from build123d import *

# Parameters (mm, degrees)
SKETCH1_W              = 36
SKETCH1_H              = 79.20150733
BOSS_EXTRUDE1_DEPTH    = 33.93
CUT_EXTRUDE1_REACH     = 65.368
SKETCH2_W              = 23.93
SKETCH2_H              = 8
SKETCH3_W              = 30.4
SKETCH3_H              = 7.2
CUT_EXTRUDE2_DEPTH     = 31.93
CUT_EXTRUDE3_START     = -3
CUT_EXTRUDE3_DEPTH     = 73.2
CUT_EXTRUDE4_REACH     = 55.961
BOSS_EXTRUDE2_REACH    = 57.168
LPATTERN1_COUNT        = 4
LPATTERN1_PITCH        = 16.8
LPATTERN1_COPY_1_REACH = 57.168
LPATTERN1_COPY_2_REACH = 57.168
LPATTERN1_COPY_3_REACH = 57.168
SKETCH7_W              = 36
SKETCH7_H              = 79.20150733
CUT_EXTRUDE5_DEPTH     = 2
FILLET1_R              = 1.5875
MOVE_START             = -34.93
MOVE_FACE1_OUTLINE_W   = 36
MOVE_FACE1_OUTLINE_H   = 63.20150733
MOVE_FACE1_DEPTH       = 1


# Read off the part's stored shape, not the designer's step: Move Face1
with BuildPart() as part:
    # Sketch1 → Boss-Extrude1 (new body)
    with BuildSketch(Plane.XY):
        Rectangle(SKETCH1_W, SKETCH1_H)
    extrude(amount=-BOSS_EXTRUDE1_DEPTH)

    # Sketch2 → Cut-Extrude1 (cut, up to next)
    with BuildSketch(Plane(origin=(18, 0, 0), x_dir=(0, 0, -1), z_dir=(1, 0, 0)), mode=Mode.PRIVATE) as cut_extrude1_sk1:
        with Locations((21.965, 35.600753665)):
            Rectangle(SKETCH2_W, SKETCH2_H)
    cut_extrude1_tool1 = extrude(cut_extrude1_sk1.sketch, amount=-CUT_EXTRUDE1_REACH, mode=Mode.PRIVATE) & part.part
    # Sketch2 → Cut-Extrude1 (cut, up to next)
    with BuildSketch(Plane(origin=(18, 0, 0), x_dir=(0, 0, -1), z_dir=(1, 0, 0)), mode=Mode.PRIVATE) as cut_extrude1_sk2:
        with Locations((21.965, -35.600753665)):
            Rectangle(SKETCH2_W, SKETCH2_H)
    cut_extrude1_tool2 = extrude(cut_extrude1_sk2.sketch, amount=-CUT_EXTRUDE1_REACH, mode=Mode.PRIVATE) & part.part
    add(cut_extrude1_tool1.solids().sort_by_distance((18, 35.600754, -21.965))[0], mode=Mode.SUBTRACT)
    add(cut_extrude1_tool2.solids().sort_by_distance((18, -35.600754, -21.965))[0], mode=Mode.SUBTRACT)

    # Sketch3 → Cut-Extrude2 (cut)
    with BuildSketch(Plane.XY):
        with Locations((0, 8.400251222)):
            Rectangle(SKETCH3_W, SKETCH3_H)
        with Locations((0, 25.200753665)):
            Rectangle(SKETCH3_W, SKETCH3_H)
        with Locations((0, -8.400251222)):
            Rectangle(SKETCH3_W, SKETCH3_H)
        with Locations((0, -25.200753665)):
            Rectangle(SKETCH3_W, SKETCH3_H)
    extrude(amount=-CUT_EXTRUDE2_DEPTH, mode=Mode.SUBTRACT)

    # Sketch4 → Cut-Extrude3 (cut)
    with BuildSketch(Plane(origin=(0, 39.600753665, 0), x_dir=(1, 0, 0), z_dir=(0, 1, 0)).offset(CUT_EXTRUDE3_START)):
        Polygon((-8, 0), (0, 5), (8, 0), align=None)
    extrude(amount=-CUT_EXTRUDE3_DEPTH, mode=Mode.SUBTRACT)

    # Sketch5 → Cut-Extrude4 (cut, up to next)
    with BuildSketch(Plane.XY.offset(-31.93), mode=Mode.PRIVATE) as cut_extrude4_sk1:
        with BuildLine():
            Line((-2.89, 26.780753665), (2.89, 26.780753665))
            ThreePointArc((2.89, 26.780753665), (4.47, 25.200753665), (2.89, 23.620753665))
            Line((2.89, 23.620753665), (-2.89, 23.620753665))
            ThreePointArc((-2.89, 23.620753665), (-4.47, 25.200753665), (-2.89, 26.780753665))
        make_face()
    cut_extrude4_tool1 = extrude(cut_extrude4_sk1.sketch, amount=-CUT_EXTRUDE4_REACH, mode=Mode.PRIVATE) & part.part
    cut_extrude4 = cut_extrude4_tool1.solids().sort_by_distance((0, 25.200754, -31.93))[0]
    add(cut_extrude4, mode=Mode.SUBTRACT)

    # Sketch6 → Boss-Extrude2 (add, up to next)
    with BuildSketch(Plane.XY, mode=Mode.PRIVATE) as boss_extrude2_sk1:
        Polygon((-15.2, 25.423123011), (-15.2, 24.450753665), (-14.7, 24.450753665), (-14.7, 24.896968819), align=None)
    boss_extrude2_tool1 = extrude(boss_extrude2_sk1.sketch, amount=-BOSS_EXTRUDE2_REACH, mode=Mode.PRIVATE) - part.part
    boss_extrude2 = boss_extrude2_tool1.solids().sort_by_distance((-14.980908, 24.821662, 0))[0]
    add(boss_extrude2)

    # Mirror1: Boss-Extrude2 across plane
    add(boss_extrude2.mirror(Plane(origin=(0, 0, 0), x_dir=(0, 0, 1), z_dir=(1, 0, 0))))

    # LPattern1: Cut-Extrude4, Boss-Extrude2 ×4
    with Locations(*[(0, -i * LPATTERN1_PITCH, 0) for i in range(1, LPATTERN1_COUNT)]):
        add(cut_extrude4, mode=Mode.SUBTRACT)
        add(boss_extrude2)

    # LPattern1 copy 1 sketch → LPattern1 copy 1 (add, up to next)
    with BuildSketch(Plane(origin=(0, -16.8, 0), x_dir=(-1, 0, 0), z_dir=(0, 0, 1)), mode=Mode.PRIVATE) as lpattern1_copy_1_sk1:
        Polygon((-15.2, -25.423123011), (-15.2, -24.450753665), (-14.7, -24.450753665), (-14.7, -24.896968819), align=None)
    lpattern1_copy_1_tool1 = extrude(lpattern1_copy_1_sk1.sketch, amount=-LPATTERN1_COPY_1_REACH, mode=Mode.PRIVATE) - part.part
    add(lpattern1_copy_1_tool1.solids().sort_by_distance((14.980908, 8.021662, 0))[0])

    # LPattern1 copy 2 sketch → LPattern1 copy 2 (add, up to next)
    with BuildSketch(Plane(origin=(0, -33.6, 0), x_dir=(-1, 0, 0), z_dir=(0, 0, 1)), mode=Mode.PRIVATE) as lpattern1_copy_2_sk1:
        Polygon((-15.2, -25.423123011), (-15.2, -24.450753665), (-14.7, -24.450753665), (-14.7, -24.896968819), align=None)
    lpattern1_copy_2_tool1 = extrude(lpattern1_copy_2_sk1.sketch, amount=-LPATTERN1_COPY_2_REACH, mode=Mode.PRIVATE) - part.part
    add(lpattern1_copy_2_tool1.solids().sort_by_distance((14.980908, -8.778338, 0))[0])

    # LPattern1 copy 3 sketch → LPattern1 copy 3 (add, up to next)
    with BuildSketch(Plane(origin=(0, -50.4, 0), x_dir=(-1, 0, 0), z_dir=(0, 0, 1)), mode=Mode.PRIVATE) as lpattern1_copy_3_sk1:
        Polygon((-15.2, -25.423123011), (-15.2, -24.450753665), (-14.7, -24.450753665), (-14.7, -24.896968819), align=None)
    lpattern1_copy_3_tool1 = extrude(lpattern1_copy_3_sk1.sketch, amount=-LPATTERN1_COPY_3_REACH, mode=Mode.PRIVATE) - part.part
    add(lpattern1_copy_3_tool1.solids().sort_by_distance((14.980908, -25.578338, 0))[0])

    # Sketch7 → Cut-Extrude5 (cut)
    with BuildSketch(Plane.XY):
        Rectangle(SKETCH7_W, SKETCH7_H)
        Polygon((-15.2, -36.599246335), (15.2, -36.599246335), (15.2, -25.949246335), (14.7, -25.949246335), (14.7, -25.503031181), (15.2, -24.976876989), (15.2, -9.149246335), (14.7, -9.149246335), (14.7, -8.703031181), (15.2, -8.176876989), (15.2, 7.650753665), (14.7, 7.650753665), (14.7, 8.096968819), (15.2, 8.623123011), (15.2, 24.450753665), (14.7, 24.450753665), (14.7, 24.896968819), (15.2, 25.423123011), (15.2, 36.600753665), (-15.2, 36.600753665), (-15.2, 25.423123011), (-14.7, 24.896968819), (-14.7, 24.450753665), (-15.2, 24.450753665), (-15.2, 8.623123011), (-14.7, 8.096968819), (-14.7, 7.650753665), (-15.2, 7.650753665), (-15.2, -8.176876989), (-14.7, -8.703031181), (-14.7, -9.149246335), (-15.2, -9.149246335), (-15.2, -24.976876989), (-14.7, -25.503031181), (-14.7, -25.949246335), (-15.2, -25.949246335), align=None, mode=Mode.SUBTRACT)
    extrude(amount=-CUT_EXTRUDE5_DEPTH, mode=Mode.SUBTRACT)

    # Fillet1
    fillet1_edges = [part.edges().sort_by_distance(p)[0] for p in [
        (15.2, 36.600753665, -1),
        (-15.2, -36.599246335, -1),
        (-15.2, 36.600753665, -1),
        (15.2, -36.599246335, -1),
    ]]
    fillet(fillet1_edges, radius=FILLET1_R)

    # Move Face1 outline → Move Face1 (add)
    with BuildSketch(Plane.XY.offset(MOVE_START)):
        Rectangle(MOVE_FACE1_OUTLINE_W, MOVE_FACE1_OUTLINE_H)
        with BuildLine():
            ThreePointArc((-2.89, -26.779246335), (-4.47, -25.199246335), (-2.89, -23.619246335))
            Line((-2.89, -23.619246335), (2.89, -23.619246335))
            ThreePointArc((2.89, -23.619246335), (4.47, -25.199246335), (2.89, -26.779246335))
            Line((2.89, -26.779246335), (-2.89, -26.779246335))
        make_face(mode=Mode.SUBTRACT)
        with BuildLine():
            ThreePointArc((-2.89, -9.979246335), (-4.47, -8.399246335), (-2.89, -6.819246335))
            Line((-2.89, -6.819246335), (2.89, -6.819246335))
            ThreePointArc((2.89, -6.819246335), (4.47, -8.399246335), (2.89, -9.979246335))
            Line((2.89, -9.979246335), (-2.89, -9.979246335))
        make_face(mode=Mode.SUBTRACT)
        with BuildLine():
            ThreePointArc((-2.89, 6.820753665), (-4.47, 8.400753665), (-2.89, 9.980753665))
            Line((-2.89, 9.980753665), (2.89, 9.980753665))
            ThreePointArc((2.89, 9.980753665), (4.47, 8.400753665), (2.89, 6.820753665))
            Line((2.89, 6.820753665), (-2.89, 6.820753665))
        make_face(mode=Mode.SUBTRACT)
        with BuildLine():
            ThreePointArc((-2.89, 23.620753665), (-4.47, 25.200753665), (-2.89, 26.780753665))
            Line((-2.89, 26.780753665), (2.89, 26.780753665))
            ThreePointArc((2.89, 26.780753665), (4.47, 25.200753665), (2.89, 23.620753665))
            Line((2.89, 23.620753665), (-2.89, 23.620753665))
        make_face(mode=Mode.SUBTRACT)
    extrude(amount=MOVE_FACE1_DEPTH)


solid = part.part
Build history of the part. All positions in model axes, mm. A direction names the side the tool comes from. Give positions to 0.01 mm unless a question says otherwise; leave off trailing zeros. Order: outer loops, then holes, each group sorted by start corner. A loop starts at its lowest first (then second) coordinate and runs counter-clockwise, first axis right, second up. Notation, with made-up numbers: M -3.75,67.25 L 32.25,67.25 A10 ccw 32.25,79.25 Z; hole C 65,-15 d3. An arc over 180 degrees is marked long. Put each result on its own line as item: value.
Item 1: Pull direction Y, two halves, no side cores. Call faces 4 (the face through (0, 21.601, -16)), 5 (the face through (15.2, -7, -17)), 6 (the face through (15.2, -32, -1)), 7 (the face through (-14.72, -36.15, -1.01)): +Y half, -Y half, draft (parallel to the pull), parting line (faces both ways), or undercut.
Results are:
face 4: undercut
face 5: undercut
face 6: draft
face 7: -Y half
Item 2: Cut at A-A on y = 14. Write the cut outline in (x, z).
Results are:
outline: M -18,-34.93 L 18,-34.93 L 18,-2 L 15.2,-2 L 15.2,0 L 8,0 L 0,-5 L -8,0 L -15.2,0 L -15.2,-2 L -18,-2 Z
Item 3: Cut at B-B on x = 6. Write the cut outline in (y, z).
Results are:
outline: M -39.6,-10 L -31.6,-10 L -31.6,-34.93 L 31.6,-34.93 L 31.6,-10 L 39.6,-10 L 39.6,-2 L 36.6,-2 L 36.6,-1.25 L 28.8,-1.25 L 28.8,-31.93 L 21.6,-31.93 L 21.6,-1.25 L 12,-1.25 L 12,-31.93 L 4.8,-31.93 L 4.8,-1.25 L -4.8,-1.25 L -4.8,-31.93 L -12,-31.93 L -12,-1.25 L -21.6,-1.25 L -21.6,-31.93 L -28.8,-31.93 L -28.8,-1.25 L -36.6,-1.25 L -36.6,-2 L -39.6,-2 Z
Item 4: Cut at D-D on x = -7. Write the cut outline in (y, z) (3 decimals).
Results are:
outline: M -39.601,-10 L -31.601,-10 L -31.601,-34.93 L 31.601,-34.93 L 31.601,-10 L 39.601,-10 L 39.601,-2 L 36.601,-2 L 36.601,-0.625 L 28.801,-0.625 L 28.801,-31.93 L 21.601,-31.93 L 21.601,-0.625 L 12,-0.625 L 12,-31.93 L 4.8,-31.93 L 4.8,-0.625 L -4.8,-0.625 L -4.8,-31.93 L -12,-31.93 L -12,-0.625 L -21.601,-0.625 L -21.601,-31.93 L -28.801,-31.93 L -28.801,-0.625 L -36.599,-0.625 L -36.599,-2 L -39.601,-2 Z
Item 5: Drop flat-ended pins along their axis: pin 1 Ø12 at (x, z) = (-3, -31) entering from +Y; pin 2 Ø3.5 at (x, y) = (6, -25) entering from +Z; pin 3 Ø3.5 at (x, z) = (-1, -33) entering from -Y. Give the stop position or say it passes through.
Results are:
pin 1: y = 31.6
pin 2: z = -31.93
pin 3: y = -31.6
Item 6: Cut at C-C on z = -7. Count the separate pieces of the cut face and the enclosed holes in it, then the cut area to 3 significant figures.
Results are:
separate pieces: 1
enclosed holes: 4
area: 1,980 mm2
Item 7: Wall check: probe 1 along Y at (x, z) = (-4.5, -27.5); probe 2 along X at (y, z) = (-22, -21); probe 3 along Y at (x, z) = (6, -6.5). Give the ranges that are in metal, low to high.
Results are:
probe 1: -31.6 to -28.8, -21.6 to -12, -4.8 to 4.8, 12 to 21.6, 28.8 to 31.6
probe 2: -18 to -15.2, 15.2 to 18
probe 3: -39.6 to -28.8, -21.6 to -12, -4.8 to 4.8, 12 to 21.6, 28.8 to 39.6
Item 8: Which spindle directions (+Z, -Z, +X, -X, +Y, -Y) get a long thin tool onto all of the face, cutting with end or side? Do faces 1 (the face through (-4.056, 16.868, -2.465)), 2 (the face through (4.47, 8.44, -33.45)), 3 (the face through (15.2, -17, -1)). Say none if no direction does.
Results are:
face 1: +Z
face 2: +Z, -Z
face 3: +Z, +X, +Y, -Y
